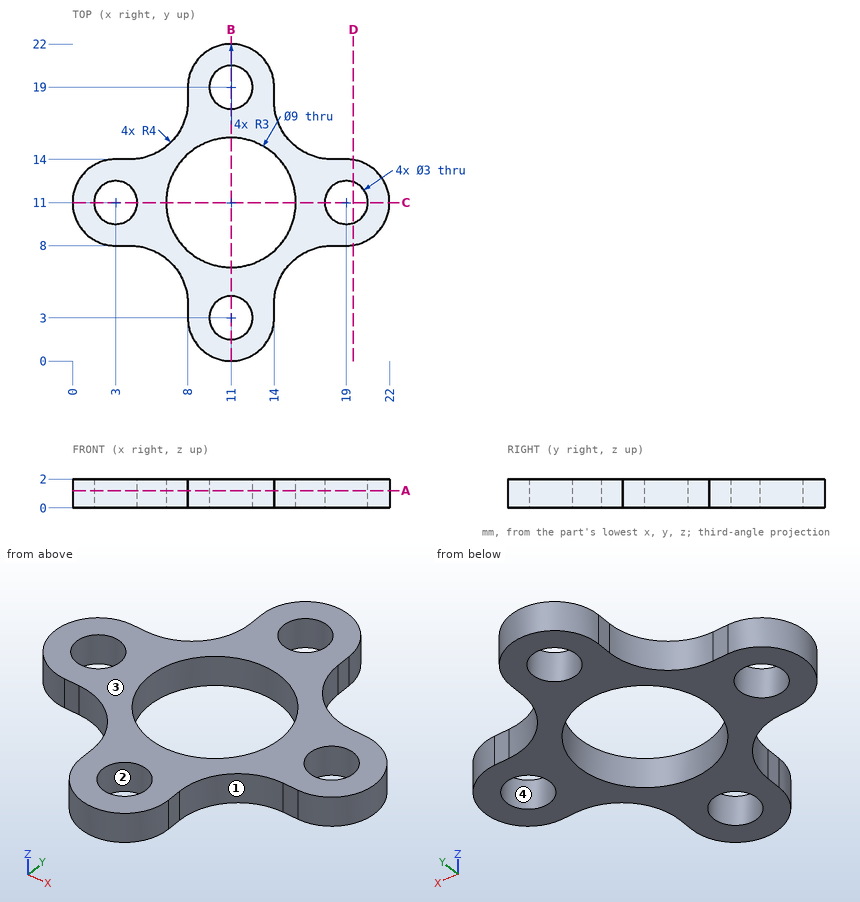
The figure shows three views and two pictorial views of one solid part (mm, origin at its lowest corner). Answer the questions. Give positions to 0.01 mm unless a question says otherwise; leave off trailing zeros. Write each loop counter-clockwise with the first axis right and the second up, starting at its lowest first coordinate (ties: lowest second). Pieces come first, ordered by that corner, then holes.
Q1. The part is cut by section A-A on z = 1.2. Give the vertices of the cut face in (x, y).
Answer:
outline: (3, 8) - (4, 8) arc R4 cw to (8, 4) - (8, 3) arc R3 ccw to (14, 3) - (14, 4) arc R4 cw to (18, 8) - (19, 8) arc R3 ccw to (19, 14) - (18, 14) arc R4 cw to (14, 18) - (14, 19) arc R3 ccw to (8, 19) - (8, 18) arc R4 cw to (4, 14) - (3, 14) arc R3 ccw to start; hole circle Ø3 at (3, 11); hole circle Ø9 at (11, 11); hole circle Ø3 at (11, 3); hole circle Ø3 at (11, 19); hole circle Ø3 at (19, 11)
Q2. For a pull along Y with two mould halves and no side action, classify the marked faces 1, 2, 3 and 4 as released by +Y, released by -Y, zero draft, split by the parting line, or undercut.
Answer:
face 1: released by -Y
face 2: undercut
face 3: zero draft
face 4: undercut
Q3. Given pin 1 (1.1 mm diameter, centred on x = 18.5, z = 0.5, fed in from -Y); pin 2 (0.8 mm diameter, centred on x = 3.5, z = 1, fed in from +Y); pin 3 (1 mm diameter, centred on x = 6.5, z = 1, fed in from -Y); pin 4 (3.5 mm diameter, centred on x = 19, y = 11, fed in from +Z), each flat-ended and moving along its own axis, determine where each tip first touches the part or whether it passes through.
Answer:
pin 1: stops at y = 8
pin 2: stops at y = 14
pin 3: stops at y = 6.65
pin 4: stops at z = 2
Q4. Straight lines are drawn through the part: L1, parallel to Y at x = 11, z = 1.55; L2, parallel to X at y = 10, z = 1.45; L3, parallel to Y at x = 19, z = 0.8. For each, find the intervals that lie inside material, in ascending order.
Answer:
L1: y = 0 to 1.5, 4.5 to 6.5, 15.5 to 17.5, 20.5 to 22
L2: x = 0.17 to 1.88, 4.12 to 6.61, 15.39 to 17.88, 20.12 to 21.83
L3: y = 8 to 9.5, 12.5 to 14
Q5. The part is cut by section D-D on x = 19.5. Give the vertices of the cut face in (y, z).
Answer:
outline: (8.04, 0) - (9.59, 0) - (9.59, 2) - (8.04, 2) - close; (12.41, 0) - (13.96, 0) - (13.96, 2) - (12.41, 2) - close
Q6. The part is cut by section B-B on x = 11. Give the vertices of the cut face in (y, z), and give its area (3 significant figures).
Answer:
outline: (0, 0) - (1.5, 0) - (1.5, 2) - (0, 2) - close; (4.5, 0) - (6.5, 0) - (6.5, 2) - (4.5, 2) - close; (15.5, 0) - (17.5, 0) - (17.5, 2) - (15.5, 2) - close; (20.5, 0) - (22, 0) - (22, 2) - (20.5, 2) - close
area: 14.0 mm2
